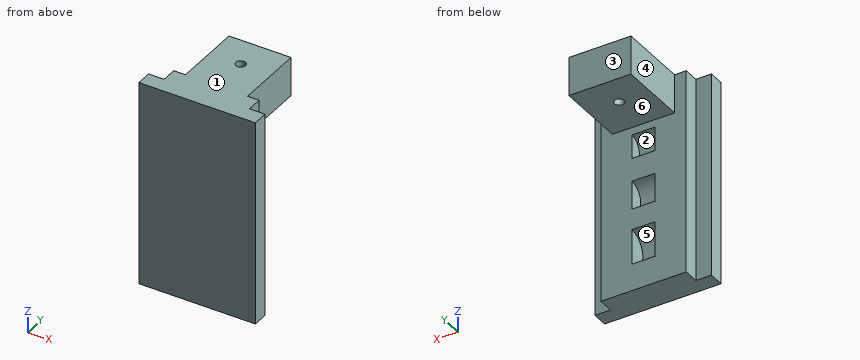
from build123d import *

# Parameters (mm, degrees)
EXTRUDE_1_DEPTH     = 6
EXTRUDE_2_DEPTH     = 52.819277108
EXTRUDE_3_DEPTH     = 52.819277108
SKETCH_6_W          = 16
SKETCH_6_H          = 10
EXTRUDE_5_DEPTH     = 18
SKETCH_7_R          = 1.25
CUT_EXTRUDE_2_DEPTH = 10


with BuildPart() as part:
    # Эскиз1 → Бобышка-Вытянуть1 (new body)
    with BuildSketch(Plane(origin=(0, 0, 0), x_dir=(0, 0, -1), z_dir=(1, 0, 0))):
        with BuildLine():
            Line((0, 0), (52.819277108, 0))
            Line((52.819277108, 0), (52.819277108, 8))
            Line((52.819277108, 8), (45.879518072, 8))
            ThreePointArc((45.879518072, 8), (41.34939759, 3.469879518), (36.819277108, 8))
            Line((36.819277108, 8), (31.421686747, 8))
            ThreePointArc((31.421686747, 8), (27.759036145, 4.337349398), (24.096385542, 8))
            Line((24.096385542, 8), (18.120481928, 8))
            ThreePointArc((18.120481928, 8), (15.036144578, 4.915662651), (11.951807229, 8))
            Line((11.951807229, 8), (0, 8))
            Line((0, 8), (0, 0))
        make_face()
    extrude(amount=EXTRUDE_1_DEPTH)

    # Эскиз2 → Бобышка-Вытянуть2 (add)
    with BuildSketch(Plane.XY):
        Polygon((6, 8), (14, 8), (14, 4), (18, 4), (18, 0), (6, 0), align=None)
    extrude(amount=-EXTRUDE_2_DEPTH)

    # Эскиз3 → Бобышка-Вытянуть3 (add)
    with BuildSketch(Plane.XY):
        Polygon((0, 8), (-8, 8), (-8, 4), (-12, 4), (-12, 0), (0, 0), align=None)
    extrude(amount=-EXTRUDE_3_DEPTH)

    # Эскиз6 → Бобышка-Вытянуть5 (add)
    with BuildSketch(Plane(origin=(0, 8, 0), x_dir=(1, 0, 0), z_dir=(0, 1, 0))):
        with Locations((3, 5)):
            Rectangle(SKETCH_6_W, SKETCH_6_H)
    extrude(amount=EXTRUDE_5_DEPTH)

    # Эскиз7 → Вырез-Вытянуть2 (cut)
    with BuildSketch(Plane.XY):
        with Locations((3, 18)):
            Circle(SKETCH_7_R)
    extrude(amount=-CUT_EXTRUDE_2_DEPTH, mode=Mode.SUBTRACT)


solid = part.part
Design review of the part built by this model. Coordinates are the model's own, in mm. Face numbers are marked on the shaded views. A direction names the side the tool comes from. Round coordinates to 2 decimals unless told otherwise and drop trailing zeros. Loops run counter-clockwise (first coordinate to the right, second up) from the corner with the lowest first, then second, coordinate; pieces in that order, holes last. Notation, with made-up numbers: M 55,-13 L 105,-13 A18 cw 105,6 Z; hole C -2,-2 d10. An arc over 180 degrees is marked long. Answer as a JSON object with one key per item and string values.
Item 1: We need section A-A on y = 18. Give the boundary of the cut face in (x, z).
Answer sheet:
{"outline": "M -5,-10 L 1.75,-10 L 1.75,0 L -5,0 Z; M 4.25,-10 L 11,-10 L 11,0 L 4.25,0 Z"}
Item 2: Clearance check with flat-ended pins moving along their axes: P1, Ø3, axis at y = 7, z = -28.5, coming from the +X side; P2, Ø4, axis at x = 3, y = 18, coming from the -Z side; P3, Ø12, axis at y = 19, z = -34.5, coming from the -X side; P4, Ø3, axis at y = 6.5, z = -23.5, coming from the -X side. State where each tip first meets the part, or that it passes through.
Answer sheet:
{"P1": "stops at x = 14", "P2": "stops at z = -10", "P3": "passes through", "P4": "stops at x = -8"}
Item 3: Wall thickness on L1, parallel to Y at x = 3, z = -5.5; L2, parallel to Z at x = -3.25, y = 23; L3, parallel to Y at x = 1.25, z = -18.5: over which ranges is each line inside the solid? List them lowest first. Write a range as from..to.
Answer sheet:
{"L1": "y = 0..16.75, 19.25..26", "L2": "z = -10..0", "L3": "y = 0..8"}
Item 4: We need section B-B on x = 3. Give the boundary of the cut face in (y, z).
Answer sheet:
{"outline": "M 0,-52.82 L 8,-52.82 L 8,-45.88 A4.53 cw 8,-36.82 L 8,-31.42 A3.66 cw 8,-24.1 L 8,-18.12 A3.08 cw 8,-11.95 L 8,-10 L 16.75,-10 L 16.75,0 L 0,0 Z; M 19.25,-10 L 26,-10 L 26,0 L 19.25,0 Z"}
Item 5: We need section D-D on y = 20.75. Give the boundary of the cut face in (x, z), and give its area (3 significant figures).
Answer sheet:
{"outline": "M -5,-10 L 11,-10 L 11,0 L -5,0 Z", "area": "160 mm^2"}
Item 6: The part is to be moulded in two halves that separate along Z. For the marked faces 1, 2 and 3, say which applies: pulls with the +Z half, pulls with the -Z half, needs draft (parallel to the pull), parting line crosses it, or undercut.
Answer sheet:
{"face 1": "pulls with the +Z half", "face 2": "undercut", "face 3": "needs draft"}
Item 7: We need section C-C on z = -40. Give the boundary of the cut face in (x, y).
Answer sheet:
{"outline": "M -12,0 L 18,0 L 18,4 L 14,4 L 14,8 L 6,8 L 6,3.68 L 0,3.68 L 0,8 L -8,8 L -8,4 L -12,4 Z"}
Item 8: Machinability: for the marked faces 4, 5 and 6, which of the approach directions +Z, -Z, +X, -X, +Y, -Y give a long, thin tool a straight path to every point of the face, cutting with its end or side? Answer none if there is none.
Answer sheet:
{"face 4": "+Z, -Z, -X, +Y", "face 5": "+Y", "face 6": "-Z, +X, -X, +Y"}
